Source: CAD feature listing. Evaluate the final solid. Frame: model axes, mm. Coordinates: 2 decimals unless noted, no trailing zeros. Loops run counter-clockwise (first coordinate to the right, second up) from the corner with the lowest first, then second, coordinate; pieces in that order, holes last. Notation, with made-up numbers: M 61.5,67.25 L 82.5,67.25 A11 ccw 82.5,85.25 Z; hole C 11,67 d3. An arc over 180 degrees is marked long. Write each question's results on one line, items separated by ' | '. Start each with the question number.
from build123d import *

# Parameters (mm, degrees)
SKETCH_1_R      = 2
EXTRUDE_1_DEPTH = 2


with BuildPart() as part:
    # 草图1 → 凸台-拉伸1 (new body, symmetric)
    with BuildSketch(Plane.XY):
        with BuildLine():
            ThreePointArc((-25.242857143, -2.321857103), (0, 10.683750346), (25.242857143, -2.321857103))
            ThreePointArc((25.242857143, -2.321857103), (30.821857103, -3.257142857), (31.757142857, 2.321857103))
            ThreePointArc((31.757142857, 2.321857103), (0, 18.683750346), (-31.757142857, 2.321857103))
            ThreePointArc((-31.757142857, 2.321857103), (-30.821857103, -3.257142857), (-25.242857143, -2.321857103))
        make_face()
        with Locations((28.5, 0)):
            Circle(SKETCH_1_R, mode=Mode.SUBTRACT)
        with Locations((-28.5, 0)):
            Circle(SKETCH_1_R, mode=Mode.SUBTRACT)
    extrude(amount=EXTRUDE_1_DEPTH, both=True)


solid = part.part
Item 1: Mould query, pull axis Y, two halves, no side actions, for faces 1 (the cylindrical face through (0.52, 18.68, 0.03)), 2 (the cylindrical face through (30.408, 0.601, -0.028)), 3 (the cylindrical face through (-0.41, 10.68, 0.03)). Classes: +Y half, -Y half, draft (parallel to the pull), parting line (faces both ways), or undercut.
Item 2: First-contact query: pin 1 Ø1 at (x, z) = (-23, 0.5) entering from +Y; pin 2 Ø1 at (x, z) = (21, -0.5) entering from +Y. Flat tips, straight axial feed; report the tip coordinate or a pass-through.
Item 3: Cut plane A-A (y = 9.75). Output: boundary loops of the cut face in (x, z).
Item 4: Cut plane B-B (x = 28.5). Output: boundary loops of the cut face in (y, z).
Item 5: Cut plane C-C (z = 0.15). Output: boundary loops of the cut face in (x, y), then the cut area to 3 significant figures.
Item 6: Cut plane D-D (y = -0.75). Output: boundary loops of the cut face in (x, z) (3 decimals), then the cut area to 3 significant figures.
Item 7: Line query: probe 1 along X at (y, z) = (8, 0.85); probe 2 along Y at (x, z) = (-28.5, 0.6); probe 3 along Y at (x, z) = (-2, 0.7). Output: solid intervals per line, ascending.
Response values:
1) face 1: +Y half | face 2: undercut | face 3: -Y half
2) pin 1: stops at y = 11.54 | pin 2: stops at y = 12.86
3) outline: M -24.84,-2 L -7.55,-2 L -7.55,2 L -24.84,2 Z; M 7.55,-2 L 24.84,-2 L 24.84,2 L 7.55,2 Z
4) outline: M -4,-2 L -2,-2 L -2,2 L -4,2 Z; M 2,-2 L 6.31,-2 L 6.31,2 L 2,2 Z
5) outline: M -31.76,2.32 A4 ccw -25.24,-2.32 A31 cw 25.24,-2.32 A4 ccw 31.76,2.32 A39 ccw Z; hole C -28.5,0 d4; hole C 28.5,0 d4 | area: 558 mm2
6) outline: M -32.429,-2 L -30.354,-2 L -30.354,2 L -32.429,2 Z; M -26.646,-2 L -24.045,-2 L -24.045,2 L -26.646,2 Z; M 24.045,-2 L 26.646,-2 L 26.646,2 L 24.045,2 Z; M 30.354,-2 L 32.429,-2 L 32.429,2 L 30.354,2 Z | area: 37.4 mm2
7) probe 1: x = -26.82 to -12.62, 12.62 to 26.82 | probe 2: y = -4 to -2, 2 to 6.31 | probe 3: y = 10.62 to 18.63
